Autodesk Inventor part; units mm, degrees
ref_plane "YZ Plane" through (0, 0, 0) normal (1, 0, 0) x (0, 1, 0)
ref_plane "XZ Plane" through (0, 0, 0) normal (0, 1, 0) x (-1, 0, 0)
ref_plane "XY Plane" through (0, 0, 0) normal (0, 0, 1) x (1, 0, 0)
sketch "Sketch1" plane through (0, 0, 0) normal (0, 1, 0) x (-1, 0, 0)
  line L0 (39.5, 16.9949) -> (118.5, 16.9949) construction
  line L1 (31.5, 10.9949) -> (39.5, 10.9949)
  line L2 (39.5, -11.0051) -> (31.5, -11.0051)
  line L3 (29.5, -10.0051) -> (31.5, -11.0051)
  line L4 (29.5, 9.9949) -> (31.5, 10.9949)
  line L5 (29.5, 9.9949) -> (29.5, -10.0051)
  line L6 (39.5, -17.0051) -> (39.5, -11.0051)
  line L7 (39.5, 10.9949) -> (39.5, 16.9949)
  line L8 (-14.5, 15) -> (15.5, 15)
  line L9 (15.5, -15) -> (-14.5, -15)
  line L10 (15.5, 15) -> (23.5, 16.9949)
  line L11 (15.5, -15) -> (23.5, -17.0051)
  line L12 (39.5, -17.0051) -> (23.5, -17.0051)
  line L13 (39.5, 16.9949) -> (23.5, 16.9949)
  line L14 (-39.5, 13) -> (-14.5, 13)
  line L15 (-39.5, -13) -> (-14.5, -13)
  line L16 (-24.5, 7) -> (-24.5, -7)
  line L17 (-24.5, 7) -> (-39.5, 7)
  line L18 (-24.5, -7) -> (-39.5, -7)
  line L19 (-39.5, 13) -> (-39.5, 7)
  line L20 (-39.5, -7) -> (-39.5, -13)
  line L21 (-17.5, 3) -> (-17.5, -3)
  line L22 (-17.5, 3) -> (-7.5, 0)
  line L23 (-7.5, 0) -> (-17.5, -3)
  line L24 (-14.5, 15) -> (-14.5, 13)
  line L25 (-14.5, -13) -> (-14.5, -15)
  line L26 (17.5, -3.0294) -> (17.5, 2.9706)
  line L27 (17.5, -3.0294) -> (7.5, -0.0294)
  line L28 (7.5, -0.0294) -> (17.5, 2.9706)
  line L29 (9.5, 7) -> (-9.5, 7)
  line L30 (0, 2) -> (9.5, 7)
  line L31 (-9.5, 7) -> (0, 2)
  line L32 (-9.5209, -7) -> (9.4791, -7)
  line L33 (-0.0209, -2) -> (-9.5209, -7)
  line L34 (9.4791, -7) -> (-0.0209, -2)
  point P0 (0, 0)
  point P1 (39.5, 13.9949)
  point P2 (-17.5, 0)
  point P3 (17.5, -0.0294)
  point P4 (-14.7945, 6.659)
  point P5 (-14.2279, -6.5477)
  point P6 (0, 7)
  point P7 (0, 7)
  dimension "d18" = 10
  dimension "d21" = 6
  dimension "d22" = 6
  dimension "d26" = 7
  dimension "d27" = 10
  dimension "d28" = 3
  dimension "d29" = 3
  dimension "d30" = 10
  dimension "d31" = 3
  dimension "d32" = 3
extrude "Extrusion1" add sketch "Sketch1" along normal blind 6
sketch "Sketch2" plane through (14.5, 0, 13) normal (0, 0, 1) x (1, 0, 0)
  line L0 (0, 6) -> (25, 6)
  line L1 (25, 0) -> (25, 6)
  circle A0 centre (23, 3) radius 1
  point P0 (-14.5, 0)
  point P1 (25, 3)
  dimension "d45" = 2
extrude "Extrusion2" cut sketch "Sketch2" against normal blind 40
sketch "Sketch3" plane through (-39.5, 0, 16.9949) normal (0, 0, 1) x (1, 0, 0)
  line L0 (8, 6) -> (0, 6)
  line L1 (0, 0) -> (0, 6)
  circle A0 centre (3.1, 3) radius 1.5
  point P0 (39.5, 0)
  dimension "d49" = 3
extrude "Extrusion3" cut sketch "Sketch3" against normal blind 40
fillet "Fillet1" radius 1 6 edges at (39.5, 3, -13) (14.5, 3, -15) (-39.5, 3, -17.0051) (39.5, 3, 13) (14.5, 3, 15) (-39.5, 3, 16.9949)
sketch "Sketch4" plane through (-15.5, 0, 15) normal (0, 0, 1) x (1, 0, 0)
  line L0 (-24, 0) -> (-24, 6)
  circle A0 centre (22, 3) radius 1
  point P0 (15.5, 0)
  dimension "d56" = 2
extrude "Extrusion4" cut sketch "Sketch4" against normal blind 8
properties part number "PX9200-10"
Read the model definition and answer for the solid it produces. Units are mm, in the model's axes. A direction names the side the tool comes from. Coordinates: 2 decimals unless noted, no trailing zeros. Order: outer loops, then holes, each group sorted by start corner. A loop starts at its lowest first (then second) coordinate and runs counter-clockwise, first axis right, second up. Notation, with made-up numbers: (55.5, -11.75) -> (66.5, -11.75) arc R11 ccw to (66.5, -1.75) -> close; hole circle Ø2 at (14, 31.5). An arc over 180 degrees is marked (long way). Answer as a JSON object with one key per item and string values.
1) Consider line 1 along X through (y, z) = (3.05, 7.5); line 2 along Z through (x, y) = (-33, 2.05); line 3 along Z through (x, y) = (26, 2.45). Determine where each line is inside the solid, lowest interval first. Write a range as from..to.
Model answer:
{"line 1": "x = -29.5..5.5, 7.5..36.5, 38.5..39.5", "line 2": "z = -17.01..-11.01, 10.99..16.99", "line 3": "z = -13..-7, 7..13"}
2) The mould has two halves that part along Y. Classify faces 1 (the face through (38.454, 3.3, -9.958)), 2 (the face through (1, 6, 0)), 3 (the face through (4.704, 2.958, -4.465)): released by +Y, released by -Y, zero draft, split by the parting line, or undercut.
Model answer:
{"face 1": "undercut", "face 2": "released by +Y", "face 3": "zero draft"}
3) A tool of negligible diameter and unlimited length cuts with its end or side. For faces 4 (the face through (12.43, 2.96, -1.48)), 5 (the face through (-29.5, 3, 0)), 6 (the face through (-1, 3, 15)), from which of +Z, -Z, +X, -X, +Y, -Y can it reach the whole face along a straight path? Write none if from no direction.
Model answer:
{"face 4": "+Y, -Y", "face 5": "-X, +Y, -Y", "face 6": "+Z, +X, +Y, -Y"}
4) A cutting plane is placed at D-D, the plane z = 1. Determine the outline of the cut face in (x, y), plus the area to 3 significant figures.
Model answer:
{"outline": "(-29.5, 0) -> (-17.5, 0) -> (-17.5, 6) -> (-29.5, 6) -> close; (-10.93, 0) -> (10.83, 0) -> (10.83, 6) -> (-10.93, 6) -> close; (17.5, 0) -> (24.5, 0) -> (24.5, 6) -> (17.5, 6) -> close", "area": "245 mm²"}
5) Each of these flat-tipped pins is pushed along its axis until it touches: pin 1 (1.8 mm diameter, centred on y = 4.5, z = 4, fed in from -X); pin 2 (0.8 mm diameter, centred on y = 4, z = 13.5, fed in from +X); pin 3 (3 mm diameter, centred on x = -36, y = 3.5, fed in from +Z); pin 4 (2.5 mm diameter, centred on x = 37.5, y = 3, fed in from -Z). Where does it stop, or does it pass through?
Model answer:
{"pin 1": "stops at x = -29.5", "pin 2": "stops at x = 14.5", "pin 3": "stops at z = 16.99", "pin 4": "stops at z = -13"}
6) A cutting plane is placed at B-B, the plane x = 16.5. Determine the outline of the cut face in (y, z).
Model answer:
{"outline": "(0, -13) -> (6, -13) -> (6, -2.7) -> (0, -2.7) -> close; (0, 2.7) -> (6, 2.7) -> (6, 13) -> (0, 13) -> close"}
7) A cutting plane is placed at C-C, the plane y = 3. State how many separate pieces and enclosed holes the cut face has, plus the area to 3 significant figures.
Model answer:
{"separate pieces": "5", "enclosed holes": "3", "area": "1,690 mm²"}
8) A cutting plane is placed at A-A, the plane x = 37.5. Determine the outline of the cut face in (y, z), plus the area to 3 significant figures.
Model answer:
{"outline": "(0, -13) -> (2, -13) -> (2, -7) -> (0, -7) -> close; (0, 7) -> (2, 7) -> (2, 13) -> (0, 13) -> close; (4, -13) -> (6, -13) -> (6, -7) -> (4, -7) -> close; (4, 7) -> (6, 7) -> (6, 13) -> (4, 13) -> close", "area": "48.0 mm²"}
